Can you work these out from the model? Positions are in its coordinate system, mm. Round coordinates to 2 decimals unless told otherwise and drop trailing zeros. Write each loop counter-clockwise with the first axis right and the second up, starting at its lowest first coordinate (ties: lowest second). Pieces come first, ordered by that corner, then holes. Notation, with made-up numbers: (22.25, 7.25) -> (41.25, 7.25) arc R25 cw to (41.25, 26.25) -> close; hole circle Ø1 at (-6, 35). An arc over 180 degrees is marked (long way). Use CSV: the item, a comma, the result in double quotes.
Autodesk Inventor part; units mm, degrees
ref_plane "Work Plane1" through (0, 31.0255, 0) normal (0, 1, 0) x (-1, 0, 0)
ref_plane "Work Plane2" through (0, 0.8255, 30.2) normal (0, 0, 1) x (1, 0, 0)
ref_plane "YZ Plane" through (0, 0, 0) normal (1, 0, 0) x (0, 1, 0)
sketch "Sketch1" plane through (0, 0, 0) normal (1, 0, 0) x (0, 1, 0)
  circle A0 centre (0.8255, 0) radius 29.2
  circle A1 centre (0.8255, 0) radius 30.2
  point P0 (0, 0)
  dimension "d0" = 58.4
  dimension "d1" = 60.4
extrude "Extrusion1" add sketch "Sketch1" along normal mid plane 60
ref_plane "Work Plane1" through (0, 31.0255, 0) normal (0, 1, 0) x (-1, 0, 0)
sketch "Sketch2" plane through (0, 31.0255, 0) normal (0, 1, 0) x (-1, 0, 0)
  line L0 (-15, -20) -> (15, -20)
  line L1 (15, -20) -> (15, 20)
  line L2 (15, 20) -> (-15, 20)
  line L3 (-15, 20) -> (-15, -20)
  line L4 (-15, -20) -> (15, 20) construction
  line L5 (15, -20) -> (-15, 20) construction
  point P0 (0, 0)
  dimension "d4" = 30
  dimension "d5" = 40
extrude "Extrusion2" cut sketch "Sketch2" against normal blind 80
ref_plane "Work Plane2" through (0, 0.8255, 30.2) normal (0, 0, 1) x (1, 0, 0)
sketch "Sketch3" plane through (0, 0.8255, 30.2) normal (0, 0, 1) x (1, 0, 0)
  circle A0 centre (0, -0.8255) radius 19.05
  dimension "d8" = 38.1
extrude "Extrusion3" cut sketch "Sketch3" against normal blind 80
properties part number "scatterBlock"
Q1. If we mould it in two halves opening along X, with no side actions, what happens to faces 1 (the face through (-30, -15, 25)), 2 (the face through (30, -15, 25)), 3 (the face through (-15, -29, 0)), 4 (the face through (15, 30.2, 0.1))? For each: released by +X, released by -X, zero draft, split by the parting line, or undercut.
Resolved:
face 1,"released by -X"
face 2,"released by +X"
face 3,"undercut"
face 4,"undercut"
Q2. Please list where these lines run through material, in increasing order: probe 1 along Y at (x, z) = (-21.5, -0.5); probe 2 along Z at (x, y) = (-1.5, -21.5); probe 3 along Y at (x, z) = (-12.5, -24.5).
Resolved:
probe 1,"y = -29.37 to -28.37, 30.02 to 31.02"
probe 2,"z = -20.34 to -20, 20 to 20.34"
probe 3,"y = -16.83 to -15.06, 16.71 to 18.48"
Q3. Will these pins go through, and if not, where does the flat tip stop? P1, Ø1.1, axis at x = -5, y = 22.5, coming from the -Z side; P2, Ø1.1, axis at x = 3, y = -21, coming from the -Z side; P3, Ø3, axis at x = 17, z = 10, coming from the -Y side.
Resolved:
P1,"stops at z = -21.58"
P2,"stops at z = -21.43"
P3,"stops at y = -28.15"
Q4. Suppose I cut it at C-C (x = -18). Write out the boundary of the cut face in (y, z), and give its area (3 significant figures).
Resolved:
outline,"(-6.24, -29.36) -> (-6.24, -28.33) arc R29.2 cw to (-6.24, 28.33) -> (-6.24, 29.36) arc R30.2 ccw to start; (6.24, -29.71) arc R30.2 ccw to (6.24, 29.71) -> (6.24, 28.69) arc R29.2 cw to (6.24, -28.69) -> close"
area,"161 mm^2"
Q5. Suppose I cut it at A-A (z = 0). Write out the boundary of the cut face in (x, y), and give its area (3 significant figures).
Resolved:
outline,"(-30, -29.37) -> (-15, -29.37) -> (-15, -28.37) -> (-30, -28.37) -> close; (-30, 30.03) -> (-15, 30.03) -> (-15, 31.03) -> (-30, 31.03) -> close; (15, -29.37) -> (30, -29.37) -> (30, -28.37) -> (15, -28.37) -> close; (15, 30.03) -> (30, 30.03) -> (30, 31.03) -> (15, 31.03) -> close"
area,"60.0 mm^2"
Q6. Suppose I cut it at B-B (x = -8.5). Write out the boundary of the cut face in (y, z), and give its area (3 significant figures).
Resolved:
outline,"(-21.8, -20) arc R30.2 ccw to (-17.05, -24.34) -> (-17.05, -23.09) arc R29.2 cw to (-20.45, -20) -> close; (-21.8, 20) -> (-20.45, 20) arc R29.2 cw to (-17.05, 23.09) -> (-17.05, 24.34) arc R30.2 ccw to start; (17.05, -25.47) arc R30.2 ccw to (23.45, -20) -> (22.1, -20) arc R29.2 cw to (17.05, -24.28) -> close; (17.05, 24.28) arc R29.2 cw to (22.1, 20) -> (23.45, 20) arc R30.2 ccw to (17.05, 25.47) -> close"
area,"26.2 mm^2"
